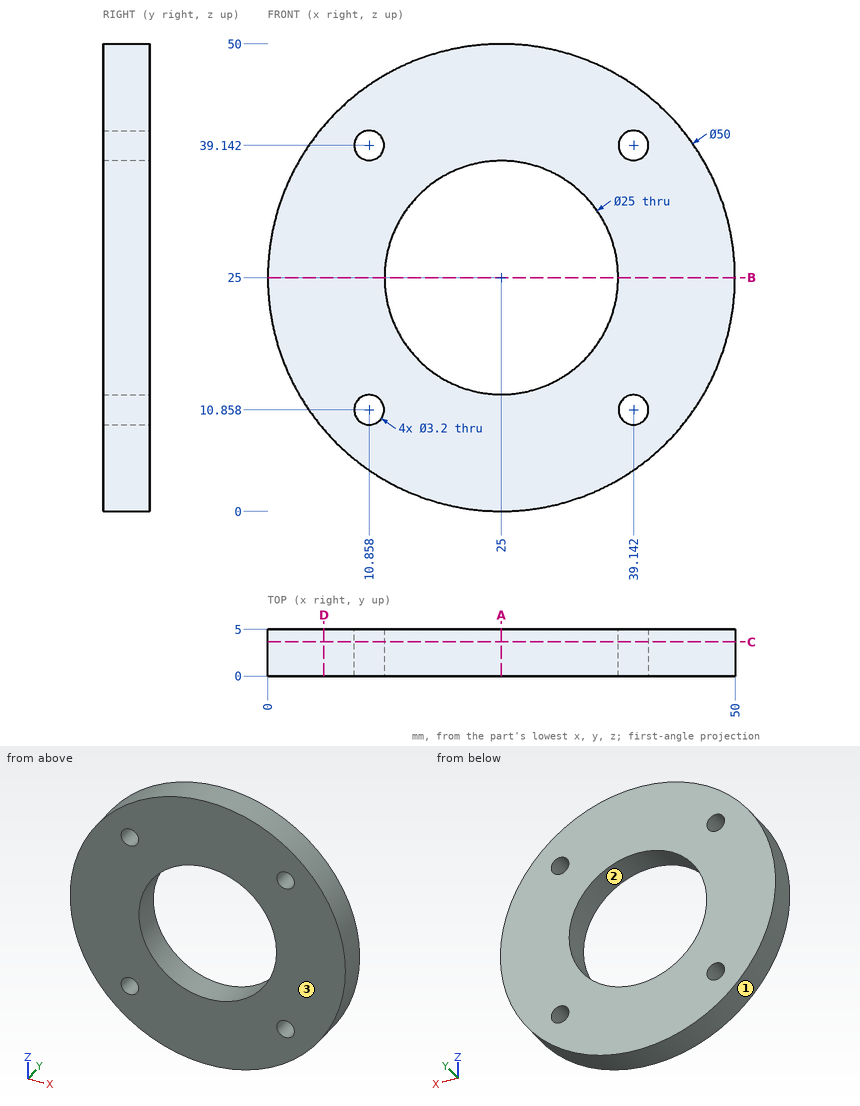
Source: three-view drawing plus pictorial views. Frame: mm from the lowest corner of the part. Give positions to 0.01 mm unless a question says otherwise; leave off trailing zeros. Order: outer loops, then holes, each group sorted by start corner. A loop starts at its lowest first (then second) coordinate and runs counter-clockwise, first axis right, second up. Notation, with made-up numbers: (-16.75, -24) -> (16.25, -24) arc R35 cw to (16.25, 12) -> close; hole circle Ø11 at (17, 8). An arc over 180 degrees is marked (long way). Put each result on its own line as item: value.
Q1. Section D-D, the plane x = 6. Return loops of the section in (y, z).
Here are the results:
outline: (0, 8.75) -> (5, 8.75) -> (5, 41.25) -> (0, 41.25) -> close
Q2. Section C-C, the plane y = 3.65. Return loops of the section in (x, z), then the cut area to 3 significant figures.
Here are the results:
outline: circle Ø50 at (25, 25); hole circle Ø3.2 at (10.86, 10.86); hole circle Ø3.2 at (10.86, 39.14); hole circle Ø25 at (25, 25); hole circle Ø3.2 at (39.14, 10.86); hole circle Ø3.2 at (39.14, 39.14)
area: 1,440 mm^2
Q3. Section A-A, the plane x = 25. Return loops of the section in (y, z), then the cut area to 3 significant figures.
Here are the results:
outline: (0, 0) -> (5, 0) -> (5, 12.5) -> (0, 12.5) -> close; (0, 37.5) -> (5, 37.5) -> (5, 50) -> (0, 50) -> close
area: 125 mm^2
Q4. Draft query along Z for the marked faces 1, 2 and 3. Return one class per face: released by +Z, released by -Z, zero draft, split by the parting line, or undercut.
Here are the results:
face 1: split by the parting line
face 2: undercut
face 3: zero draft
Q5. Section B-B, the plane z = 25. Return loops of the section in (x, y), then the cut area to 3 significant figures.
Here are the results:
outline: (0, 0) -> (12.5, 0) -> (12.5, 5) -> (0, 5) -> close; (37.5, 0) -> (50, 0) -> (50, 5) -> (37.5, 5) -> close
area: 125 mm^2
Q6. Material intervals for L1, parallel to Z at x = 25.5, y = 3.15 (3 decimals); L2, parallel to X at y = 3.05, z = 38 (1 decimal); L3, parallel to Z at x = 39, y = 4.55, sorted ascending.
Here are the results:
L1: z = 0.005 to 12.51, 37.49 to 49.995
L2: x = 3.6 to 9.7, 12 to 38, 40.3 to 46.4
L3: z = 4.29 to 9.26, 12.45 to 37.55, 40.74 to 45.71
Q7. Pin query (flat end, axial travel): pin 1 (8 mm diameter, centred on x = 11, z = 11, fed in from +Y); pin 2 (4 mm diameter, centred on x = 34, z = 23.5, fed in from +Y); pin 3 (2 mm diameter, centred on y = 3.5, z = 41.5, fed in from +X) (1 decimal). Return the tip coordinate at first contact, or that it passes through.
Here are the results:
pin 1: stops at y = 5
pin 2: passes through
pin 3: stops at x = 44.6
